```python
from build123d import *

# Parameters (mm, degrees)
F0_W        = 25
F0_H        = 25
F1_DEPTH    = 25
F2_R        = 5
F3_T1_DEPTH = 25
F3_T4_ANGLE = 90
F3_T6_ANGLE = 90


# Not quite as in the source:
# - a fillet or chamfer that OpenCascade refuses, or shapes differently, is made with other operations: its cross-section is extruded or revolved along the edge and cut away or added


with BuildPart() as f1:
    # F0 (on Top) → F1 (new body)
    with BuildSketch(Plane.XY):
        Rectangle(F0_W, F0_H)
    extrude(amount=F1_DEPTH)

    # F2
    f2_edges = [f1.edges().sort_by_distance(p)[0] for p in [
        (0, 12.5, 25),
        (-12.5, 0, 25),
        (0, -12.5, 25),
        (12.5, 0, 25),
    ]]
    fillet(f2_edges, radius=F2_R)

    # F3: fillet of radius 10 on 2 edges, made by hand

    # F3_s2 → F3_t1 (cut)
    with BuildSketch(Plane.XY):
        with BuildLine():
            ThreePointArc((12.5, -2.5), (9.5710678119, -9.5710678119), (2.5, -12.5))
            Line((2.5, -12.5), (2.5, -12.7))
            Line((2.5, -12.7), (12.7, -12.7))
            Line((12.7, -12.7), (12.7, -2.5))
            Line((12.7, -2.5), (12.5, -2.5))
        make_face()
        with BuildLine():
            ThreePointArc((-12.5, -2.5), (-9.5710678119, -9.5710678119), (-2.5, -12.5))
            Line((-2.5, -12.5), (-2.5, -12.7))
            Line((-2.5, -12.7), (-12.7, -12.7))
            Line((-12.7, -12.7), (-12.7, -2.5))
            Line((-12.7, -2.5), (-12.5, -2.5))
        make_face()
    extrude(amount=F3_T1_DEPTH, mode=Mode.SUBTRACT)

    # F3_s3 → F3_t4 (revolve, cut)
    with BuildSketch(Plane.XZ.offset(2.5)):
        with BuildLine():
            ThreePointArc((-7.5, 25), (-11.0355339059, 23.5355339059), (-12.5, 20))
            Line((-12.5, 20), (-12.5, 25))
            Line((-12.5, 25), (-7.5, 25))
        make_face()
    revolve(axis=Axis((-2.5, -2.5, 25), (0, 0, 1)), revolution_arc=F3_T4_ANGLE, mode=Mode.SUBTRACT)

    # F3_s5 → F3_t6 (revolve, cut)
    with BuildSketch(Plane.YZ.offset(2.5)):
        with BuildLine():
            ThreePointArc((-7.5, 25), (-11.0355339059, 23.5355339059), (-12.5, 20))
            Line((-12.5, 20), (-12.5, 25))
            Line((-12.5, 25), (-7.5, 25))
        make_face()
    revolve(axis=Axis((2.5, -2.5, 25), (0, 0, 1)), revolution_arc=F3_T6_ANGLE, mode=Mode.SUBTRACT)


solid = f1.part
```
Model file for the job. Use its own axes, mm. Coordinates: 2 decimals unless noted, no trailing zeros. Order: outer loops, then holes, each group sorted by start corner. A loop starts at its lowest first (then second) coordinate and runs counter-clockwise, first axis right, second up. Notation, with made-up numbers: (41, 20.25) - (92, 20.25) arc R12 ccw to (92, 30.25) - close; hole circle Ø7 at (40.25, 18). An arc over 180 degrees is marked (long way). Return JSON: item names as keys, results as strings. Group by question number.
1) Saw through at A-A, the plane z = 15.5. Write the cut outline in (x, y), plus the area to 3 significant figures.
2) Saw through at B-B, the plane y = 6.5. Write the cut outline in (x, z).
3) Probe line 1 (X direction, y = -8.75, z = 13.25); line 2 (Y direction, x = -7.75, z = 24); line 3 (X direction, y = -10, z = 22.5). List the from-to ranges inside material, lowest first. Write a range as from..to.
4) Flat gauge pin, fed straight in: P1, Ø4, axis at x = 7.5, z = 11.5, coming from the -Y side. Where does the tip first touch, or does it go through?
Values found:
{
 "1": {"outline": "(-12.5, -2.5) arc R10 ccw to (-2.5, -12.5) - (2.5, -12.5) arc R10 ccw to (12.5, -2.5) - (12.5, 12.5) - (-12.5, 12.5) - close", "area": "582 mm²"},
 "2": {"outline": "(-12.5, 0) - (12.5, 0) - (12.5, 20) arc R5 ccw to (7.5, 25) - (-7.5, 25) arc R5 ccw to (-12.5, 20) - close"},
 "3": {"line 1": "x = -10.31..10.31", "line 2": "y = -8.54..10.5", "line 3": "x = -8.05..8.05"},
 "4": {"P1": "stops at y = -12.04"}
}
